The listing builds one solid part. Answer for the finished solid, in the listing's coordinates (mm). Face numbers are marked on the shaded views. A direction names the side the tool comes from. Round coordinates to 2 decimals unless told otherwise and drop trailing zeros. Loops run counter-clockwise (first coordinate to the right, second up) from the corner with the lowest first, then second, coordinate; pieces in that order, holes last. Notation, with made-up numbers: (23.25, 70) - (44.25, 70) arc R10 cw to (44.25, 74) - close; hole circle Ø8 at (40.25, 56). An arc over 180 degrees is marked (long way). One line per question, with ' | ' between items. Start each with the question number.
from build123d import *

# Parameters (mm, degrees)
BOSS_EXTRUDE1_DEPTH      = 21
BOSS_EXTRUDE1_DEPTH_BACK = 21
SKETCH1_R                = 17.5
SKETCH1_R_2              = 12
BOSS_EXTRUDE2_DEPTH      = 9
BOSS_EXTRUDE2_DEPTH_BACK = 9
BOSS_EXTRUDE3_DEPTH      = 14
BOSS_EXTRUDE3_DEPTH_BACK = 14
SKETCH1_4_R              = 12
SKETCH1_4_R_2            = 7.5
BOSS_EXTRUDE4_DEPTH      = 2.5
BOSS_EXTRUDE4_DEPTH_BACK = 2.5


with BuildPart() as part:
    # Sketch1 → Boss-Extrude1 (new, two sides: drawn at the far end of the back side and taken through both)
    with BuildSketch(Plane(origin=(0, 0, 0), x_dir=(1, 0, 0), z_dir=(0, 1, 0)).offset(-BOSS_EXTRUDE1_DEPTH_BACK)):
        with Locations(Location((93, 0, 0), (0, 0, 270))):
            Circle(SKETCH1_R)
        with Locations(Location((93, 0, 0), (0, 0, 270))):
            Circle(SKETCH1_R_2, mode=Mode.SUBTRACT)
    extrude(amount=BOSS_EXTRUDE1_DEPTH + BOSS_EXTRUDE1_DEPTH_BACK)

    # Sketch1_3 → Boss-Extrude2 (add, two sides: drawn at the far end of the back side and taken through both)
    with BuildSketch(Plane(origin=(0, 0, 0), x_dir=(1, 0, 0), z_dir=(0, 1, 0)).offset(-BOSS_EXTRUDE2_DEPTH_BACK)):
        with BuildLine():
            Line((69.203991931, 10), (-73.167840434, 10))
            ThreePointArc((-73.167840434, 10), (-77.167840434, 10.335680868), (-81.055946811, 11.333333333))
            ThreePointArc((-81.055946811, 11.333333333), (-75.219186172, 6.952386703), (-73, 0))
            ThreePointArc((-73, 0), (-75.219186172, -6.952386703), (-81.055946811, -11.333333333))
            ThreePointArc((-81.055946811, -11.333333333), (-77.167840434, -10.335680868), (-73.167840434, -10))
            Line((-73.167840434, -10), (69.203991931, -10))
            ThreePointArc((69.203991931, -10), (76.418435276, -11.110006395), (82.965538766, -14.337349398))
            ThreePointArc((82.965538766, -14.337349398), (75.5, 0), (82.965538766, 14.337349398))
            ThreePointArc((82.965538766, 14.337349398), (76.418435276, 11.110006395), (69.203991931, 10))
        make_face()
        with BuildLine():
            Line((63, -5), (-63, -5))
            ThreePointArc((-63, -5), (-68, 0), (-63, 5))
            Line((-63, 5), (63, 5))
            ThreePointArc((63, 5), (68, 0), (63, -5))
        make_face(mode=Mode.SUBTRACT)
    extrude(amount=BOSS_EXTRUDE2_DEPTH + BOSS_EXTRUDE2_DEPTH_BACK)

    # Sketch1_4 → Boss-Extrude3 (add, two sides: drawn at the far end of the back side and taken through both)
    with BuildSketch(Plane(origin=(0, 0, 0), x_dir=(1, 0, 0), z_dir=(0, 1, 0)).offset(-BOSS_EXTRUDE3_DEPTH_BACK)):
        with Locations(Location((-85, 0, 0), (0, 0, 270))):
            Circle(SKETCH1_4_R)
        with Locations(Location((-85, 0, 0), (0, 0, 270))):
            Circle(SKETCH1_4_R_2, mode=Mode.SUBTRACT)
    extrude(amount=BOSS_EXTRUDE3_DEPTH + BOSS_EXTRUDE3_DEPTH_BACK)

    # Sketch1_5 → Boss-Extrude4 (add, two sides: drawn at the far end of the back side and taken through both)
    with BuildSketch(Plane(origin=(0, 0, 0), x_dir=(1, 0, 0), z_dir=(0, 1, 0)).offset(-BOSS_EXTRUDE4_DEPTH_BACK)):
        with BuildLine():
            ThreePointArc((-63, 5), (-68, 0), (-63, -5))
            Line((-63, -5), (63, -5))
            ThreePointArc((63, -5), (68, 0), (63, 5))
            Line((63, 5), (-63, 5))
        make_face()
    extrude(amount=BOSS_EXTRUDE4_DEPTH + BOSS_EXTRUDE4_DEPTH_BACK)


solid = part.part
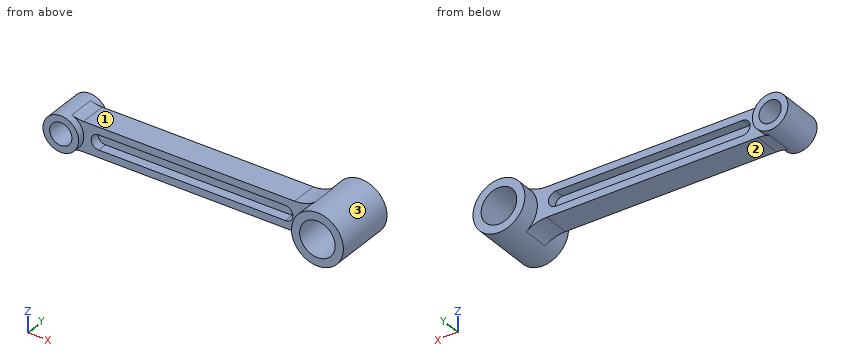
(1) Consider L1, parallel to X at y = -2, z = 0; L2, parallel to X at y = -12, z = 0; L3, parallel to X at y = -5, z = 0. Determine where each line is inside the solid, lowest interval first.
(2) Each of these flat-tipped pins is pushed along its axis until it touches: P1, Ø4, axis at x = -62.5, y = 11.5, coming from the +Z side; P2, Ø5, axis at x = -15, z = 1.5, coming from the +Y side; P3, Ø4, axis at x = 80.5, y = 1, coming from the -Z side; P4, Ø2, axis at x = -17.5, y = -7, coming from the -Z side. Where does it stop, or does it pass through?
(3) A tool of negligible diameter and unlimited length cuts with its end or side. For the marked faces 1, 2 and 3, from which of +Z, -Z, +X, -X, +Y, -Y can it reach the whole face along a straight path? Write none if from no direction.
(4) Find section D-D on x = -85. Write down the section's boundary in (y, z), plus the area to 3 significant figures.
(5) Find section A-A on x = 93. Write down the section's boundary in (y, z), plus the area to 3 significant figures.
(6) Find section B-B on z = 0. Write down the section's boundary in (x, y).
(7) Find section C-C on x = 9. Write down the section's boundary in (y, z), plus the area to 3 significant figures.
Answer below:
1) L1: -97 to -92.5, -77.5 to 81, 105 to 110.5 | L2: -97 to -92.5, -77.5 to -73, 75.5 to 81, 105 to 110.5 | L3: -97 to -92.5, -77.5 to -68, 68 to 81, 105 to 110.5
2) P1: through | P2: y = 2.5 | P3: z = -14.02 | P4: z = -10
3) face 1: +Z, +Y, -Y | face 2: -Z, +Y, -Y | face 3: none
4) outline: (-14, -12) - (14, -12) - (14, -7.5) - (-14, -7.5) - close; (-14, 7.5) - (14, 7.5) - (14, 12) - (-14, 12) - close | area: 252 mm2
5) outline: (-21, -17.5) - (21, -17.5) - (21, -12) - (-21, -12) - close; (-21, 12) - (21, 12) - (21, 17.5) - (-21, 17.5) - close | area: 462 mm2
6) outline: (-97, -14) - (-92.5, -14) - (-92.5, 14) - (-97, 14) - close; (-77.5, -14) - (-73, -14) - (-73, -9) - (-68, -9) - (-68, -2.5) - (68, -2.5) - (68, -9) - (75.5, -9) - (75.5, -21) - (81, -21) - (81, 21) - (75.5, 21) - (75.5, 9) - (68, 9) - (68, 2.5) - (-68, 2.5) - (-68, 9) - (-73, 9) - (-73, 14) - (-77.5, 14) - close; (105, -21) - (110.5, -21) - (110.5, 21) - (105, 21) - close
7) outline: (-9, -10) - (9, -10) - (9, -5) - (2.5, -5) - (2.5, 5) - (9, 5) - (9, 10) - (-9, 10) - (-9, 5) - (-2.5, 5) - (-2.5, -5) - (-9, -5) - close | area: 230 mm2
